Geometry: see drawing. Coordinates: mm, zero at the bounding-box minimum. A direction names the side the tool comes from. Give positions to 0.01 mm unless a question says otherwise; leave off trailing zeros. Write each loop counter-clockwise with the first axis right and the second up, starting at its lowest first coordinate (ties: lowest second). Pieces come first, ordered by that corner, then holes. Notation, with made-up numbers: (6, -6.5) -> (38, -6.5) arc R16 ccw to (38, 14.5) -> close; hole circle Ø1 at (1, -17). An arc over 180 degrees is marked (long way). Write item = value, one per line.
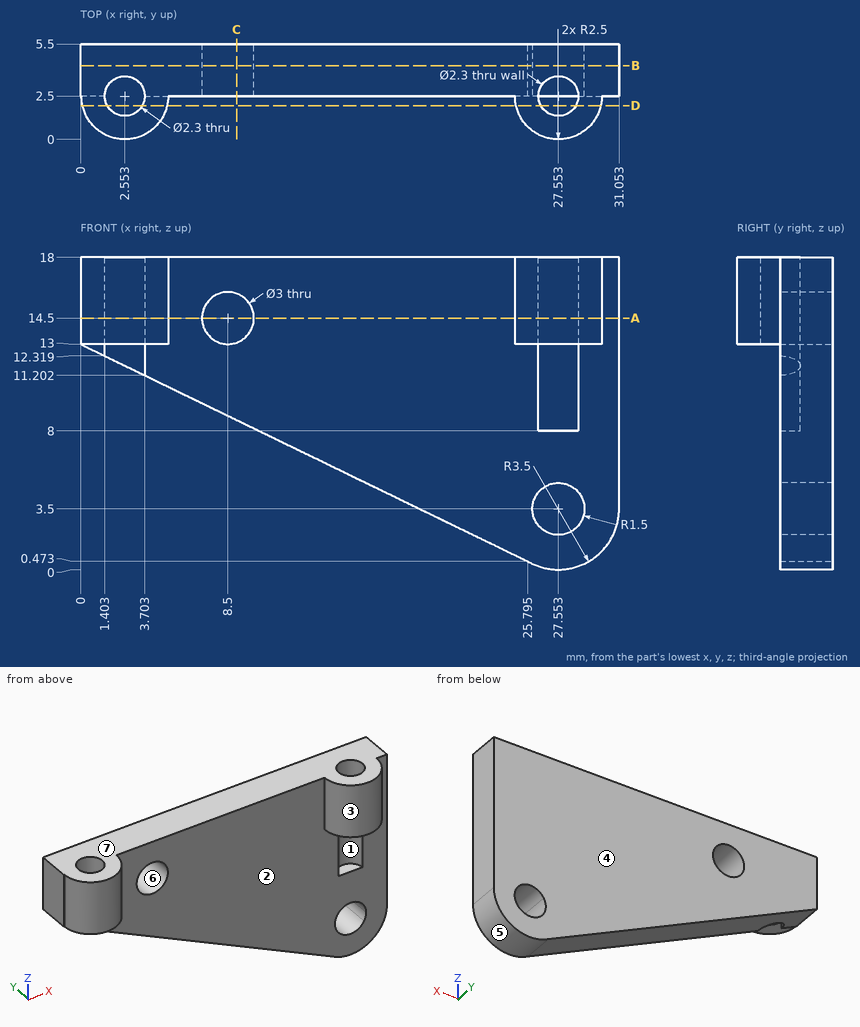
(1) Section query A-A (z = 14.5). Return loops of the section in (x, y).
Values follow:
outline = (0, 2.5) -> (0.05, 2.5) arc R2.5 ccw to (5.05, 2.5) -> (7, 2.5) -> (7, 5.5) -> (0, 5.5) -> close; (10, 2.5) -> (25.05, 2.5) arc R2.5 ccw to (30.05, 2.5) -> (31.05, 2.5) -> (31.05, 5.5) -> (10, 5.5) -> close; hole circle Ø2.3 at (2.55, 2.5); hole circle Ø2.3 at (27.55, 2.5)
(2) Material intervals for line 1 (X direction, y = 1.85, z = 15.5) (1 decimal); line 2 (Y direction, x = 29, z = 2.5); line 3 (X direction, y = 2.95, z = 16.75) (1 decimal), sorted ascending.
Values follow:
line_1 = 0.1 to 1.6, 3.5 to 5, 25.1 to 26.6, 28.5 to 30
line_2 = 2.5 to 5.5
line_3 = 0 to 1.5, 3.6 to 26.5, 28.6 to 31.1
(3) Pull-direction query (Z, two-part tool) for the marked faces 4, 5, 6 and 7; classes: pulls with the +Z half, pulls with the -Z half, needs draft (parallel to the pull), parting line crosses it, or undercut.
Values follow:
face_4 = needs draft
face_5 = pulls with the -Z half
face_6 = undercut
face_7 = pulls with the +Z half
(4) Section query C-C (x = 9). Return loops of the section in (y, z) (1 decimal), plus the area to 3 significant figures.
Values follow:
outline = (2.5, 8.6) -> (5.5, 8.6) -> (5.5, 13.1) -> (2.5, 13.1) -> close; (2.5, 15.9) -> (5.5, 15.9) -> (5.5, 18) -> (2.5, 18) -> close
area = 19.6 mm2
(5) Section query B-B (y = 4.25). Give the number of separate pieces and of enclosed holes in the cut face, plus the area to 3 significant figures.
Values follow:
separate_pieces = 1
enclosed_holes = 2
area = 368 mm2
(6) First-contact query: pin 1 (1.5 mm diameter, centred on y = 4.5, z = 5.5, fed in from -X); pin 2 (5 mm diameter, centred on x = 8.5, z = 14.5, fed in from -Y); pin 3 (1.5 mm diameter, centred on x = 20, y = 5, fed in from -Z); pin 4 (1.4 mm diameter, centred on x = 2.55, y = 2.5, fed in from -Z). Flat tips, straight axial feed; report the tip coordinate or a pass-through.
Values follow:
pin_1 = 13.9
pin_2 = 2.5
pin_3 = 2.92
pin_4 = through
(7) Access query for the marked faces 1, 2 and 3. Directions: +Z, -Z, +X, -X, +Y, -Y. A direction counts if a zero-diameter tool reaches every point of the face in a straight line with its end or side. Return the directions, or none.
Values follow:
face_1 = +Z
face_2 = -Z, -Y
face_3 = +Z, -Z, -Y
(8) Section query D-D (y = 1.95). Return loops of the section in (x, z).
Values follow:
outline = (0.11, 13) -> (1.54, 13) -> (1.54, 18) -> (0.11, 18) -> close; (3.56, 13) -> (4.99, 13) -> (4.99, 18) -> (3.56, 18) -> close; (25.11, 13) -> (26.54, 13) -> (26.54, 18) -> (25.11, 18) -> close; (28.56, 13) -> (29.99, 13) -> (29.99, 18) -> (28.56, 18) -> close
